Here's the drawing with two shaded views (mm, measured from the low corner). I have some questions. A direction names the side the tool comes from. Give positions to 0.01 mm unless a question says otherwise; leave off trailing zeros. Write each loop counter-clockwise with the first axis right and the second up, starting at its lowest first coordinate (ties: lowest second). Pieces come first, ordered by that corner, then holes.
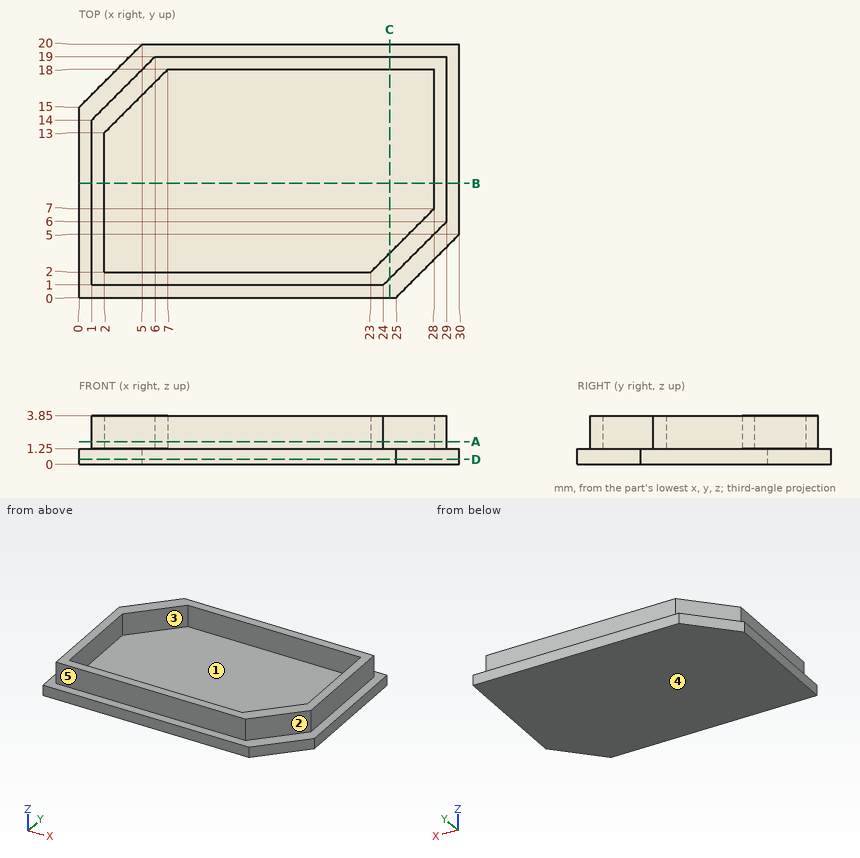
(1) Imagine slicing it at C-C, the plane x = 24.5. Write out the boundary of the cut face in (y, z), plus the area to 3 significant figures.
Returned:
outline: (0, 0) - (20, 0) - (20, 1.25) - (19, 1.25) - (19, 3.85) - (18, 3.85) - (18, 1.25) - (3.5, 1.25) - (3.5, 3.85) - (1.5, 3.85) - (1.5, 1.25) - (0, 1.25) - close
area: 32.8 mm2
(2) Imagine slicing it at D-D, the plane z = 0.4. Write out the boundary of the cut face in (x, y), plus the area to 3 significant figures.
Returned:
outline: (0, 0) - (25, 0) - (30, 5) - (30, 20) - (5, 20) - (0, 15) - close
area: 575 mm2
(3) For the marked faces 1 and 2, which set-ups out of +Z, -Z, +X, -X, +Y, -Y let a thin tool reach every point of the face, with its end or its side?
Returned:
face 1: +Z
face 2: +Z, +X, -Y
(4) Imagine slicing it at A-A, the plane z = 1.8. Write out the boundary of the cut face in (x, y), plus the area to 3 significant figures.
Returned:
outline: (1, 1) - (24, 1) - (29, 6) - (29, 19) - (6, 19) - (1, 14) - close; hole (2, 2) - (23, 2) - (28, 7) - (28, 18) - (7, 18) - (2, 13) - close
area: 88.0 mm2
(5) Will these pins go through, and if not, where does the flat tip stop? P1, Ø1.3, axis at x = 10, z = 2, coming from the +Y side; P2, Ø1.3, axis at x = 20, z = 2.5, coming from the -Y side; P3, Ø1.3, axis at y = 13, z = 2, coming from the +X side.
Returned:
P1: stops at y = 19
P2: stops at y = 1
P3: stops at x = 29
(6) Imagine slicing it at B-B, the plane y = 9. Write out the boundary of the cut face in (x, z), plus the area to 3 significant figures.
Returned:
outline: (0, 0) - (30, 0) - (30, 1.25) - (29, 1.25) - (29, 3.85) - (28, 3.85) - (28, 1.25) - (2, 1.25) - (2, 3.85) - (1, 3.85) - (1, 1.25) - (0, 1.25) - close
area: 42.7 mm2
(7) If I drill on L1, parallel to X at y = 12, z = 1.5; L2, parallel to Y at x = 18.75, z = 3.3; L3, parallel to Z at x = 12, y = 12.25, over which ranges is the centre line in solid material (lowest first)?
Returned:
L1: x = 1 to 2, 28 to 29
L2: y = 1 to 2, 18 to 19
L3: z = 0 to 1.25
(8) If we mould it in two halves opening along Y, with no side actions, what happens to the marked faces 3, 4 and 5? For each: +Y half, -Y half, draft (parallel to the pull), parting line (faces both ways), or undercut.
Returned:
face 3: undercut
face 4: draft
face 5: -Y half
